Here's how the part is built. I have some questions about the finished solid (model axes, mm). A direction names the side the tool comes from. Round coordinates to 2 decimals unless told otherwise and drop trailing zeros. Order: outer loops, then holes, each group sorted by start corner. A loop starts at its lowest first (then second) coordinate and runs counter-clockwise, first axis right, second up. Notation, with made-up numbers: M -16,-30 L -7,-30 A19 ccw -7,-5 Z; hole C -37.5,64 d2. An arc over 180 degrees is marked long. Write item = value, one per line. Start each with the question number.
Item 1: I want a section at D-D, the plane z = -4.5. List the corners of the cut face in (x, y) for me.
Item 2: I'm going to push flat-ended pins straight in: P1, Ø9, axis at x = 20.5, y = 43, coming from the -Z side; P2, Ø8.5, axis at y = 51, z = -13.5, coming from the -X side. Where does each tip first touch, or does it pass through?
Item 3: Please list where these lines run through material, in increasing order: L1, parallel to Y at x = 21, z = -2; L2, parallel to Y at x = 10, z = -1.6; L3, parallel to X at y = 52, z = -13.
Item 4: We'd pull the mould along X, two halves only. Please class faces 3 (the face through (33, 34, -10)), 4 (the face through (22.57, 17.35, -1.48)), 5 (the face through (22.57, 49.35, -1.48)), 6 (the face through (32, 34, -20)): pulls with the +X half, pulls with the -X half, needs draft (parallel to the pull), parting line crosses it, or undercut.
Item 5: For faces 1 (the face through (0, 34, -1)), 2 (the face through (15, 34, -3)), which set-ups out of +Z, -Z, +X, -X, +Y, -Y let a thin tool reach every point of the face, with its end or its side?
Item 6: I want a section at B-B, the plane y = 18. List the corners of the cut face in (x, z) for me, plus the area to 3 significant figures.
Item 7: I want a section at C-C, the plane y = 11. List the corners of the cut face in (x, z) for me.
Item 8: I want a section at A-A, the plane x = 21. List the corners of the cut face in (y, z) for me.
```python
from build123d import *

# Parameters (mm, degrees)
SKETCH_1_W          = 30
SKETCH_1_H          = 3
EXTRUDE_1_DEPTH     = 68
CUT_EXTRUDE_1_REACH = 80.186
SKETCH_2_R          = 1.7


with BuildPart() as part:
    # 草图1 → 凸台-拉伸1 (new body)
    with BuildSketch(Plane(origin=(0, 0, 0), x_dir=(1, 0, 0), z_dir=(0, 1, 0))):
        with Locations((15, 1.5)):
            Rectangle(SKETCH_1_W, SKETCH_1_H)
        Polygon((33, 20), (30, 20), (30, 3), (30, 0), (33, 0), align=None)
    extrude(amount=EXTRUDE_1_DEPTH)

    # 草图2 → 切除-拉伸1 (cut, up to next)
    with BuildSketch(Plane.XY, mode=Mode.PRIVATE) as cut_extrude_1_sk1:
        with Locations((21, 18)):
            Circle(SKETCH_2_R)
    cut_extrude_1_tool1 = extrude(cut_extrude_1_sk1.sketch, amount=-CUT_EXTRUDE_1_REACH, mode=Mode.PRIVATE) & part.part
    # 草图2 → 切除-拉伸1 (cut, up to next)
    with BuildSketch(Plane.XY, mode=Mode.PRIVATE) as cut_extrude_1_sk2:
        with Locations((21, 50)):
            Circle(SKETCH_2_R)
    cut_extrude_1_tool2 = extrude(cut_extrude_1_sk2.sketch, amount=-CUT_EXTRUDE_1_REACH, mode=Mode.PRIVATE) & part.part
    # 草图2 → 切除-拉伸1 (cut, up to next)
    with BuildSketch(Plane.XY, mode=Mode.PRIVATE) as cut_extrude_1_sk3:
        with Locations((10, 26.5)):
            Circle(SKETCH_2_R)
    cut_extrude_1_tool3 = extrude(cut_extrude_1_sk3.sketch, amount=-CUT_EXTRUDE_1_REACH, mode=Mode.PRIVATE) & part.part
    # 草图2 → 切除-拉伸1 (cut, up to next)
    with BuildSketch(Plane.XY, mode=Mode.PRIVATE) as cut_extrude_1_sk4:
        with Locations((10, 41.5)):
            Circle(SKETCH_2_R)
    cut_extrude_1_tool4 = extrude(cut_extrude_1_sk4.sketch, amount=-CUT_EXTRUDE_1_REACH, mode=Mode.PRIVATE) & part.part
    add(cut_extrude_1_tool1.solids().sort_by_distance((21, 18, 0))[0], mode=Mode.SUBTRACT)
    add(cut_extrude_1_tool2.solids().sort_by_distance((21, 50, 0))[0], mode=Mode.SUBTRACT)
    add(cut_extrude_1_tool3.solids().sort_by_distance((10, 26.5, 0))[0], mode=Mode.SUBTRACT)
    add(cut_extrude_1_tool4.solids().sort_by_distance((10, 41.5, 0))[0], mode=Mode.SUBTRACT)


solid = part.part
```
Filled in:
q1.outline = M 30,0 L 33,0 L 33,68 L 30,68 Z
q2.P1 = -3
q2.P2 = 30
q3.L1 = 0 to 16.3, 19.7 to 48.3, 51.7 to 68
q3.L2 = 0 to 24.8, 28.2 to 39.8, 43.2 to 68
q3.L3 = 30 to 33
q4.face_3 = pulls with the +X half
q4.face_4 = undercut
q4.face_5 = undercut
q4.face_6 = needs draft
q5.face_1 = +Z, -Z, -X, +Y, -Y
q5.face_2 = -Z, -X, +Y, -Y
q6.outline = M 0,-3 L 19.3,-3 L 19.3,0 L 0,0 Z; M 22.7,-3 L 30,-3 L 30,-20 L 33,-20 L 33,0 L 22.7,0 Z
q6.area = 140 mm^2
q7.outline = M 0,-3 L 30,-3 L 30,-20 L 33,-20 L 33,0 L 0,0 Z
q8.outline = M 0,-3 L 16.3,-3 L 16.3,0 L 0,0 Z; M 19.7,-3 L 48.3,-3 L 48.3,0 L 19.7,0 Z; M 51.7,-3 L 68,-3 L 68,0 L 51.7,0 Z
